from build123d import *

# Parameters (mm, degrees)
F0_W      = 43.450012
F0_H      = 38.1
F0_R      = 1.6
F1_DEPTH  = 8.5
F2_R      = 2.55
F3_DEPTH  = 3.2
F4_R      = 3.75
F5_DEPTH  = 8.5
F6_W      = 8.75
F6_H      = 8.75
F7_DEPTH  = 6.9
F8_W      = 25
F8_H      = 26
F9_DEPTH  = 5
F10_W     = 22
F10_H     = 3
F11_DEPTH = 9.225006


with BuildPart() as f1:
    # F0 (on Top) → F1 (new body)
    with BuildSketch(Plane.XY):
        Rectangle(F0_W, F0_H)
        with Locations((-15.875, -15.875)):
            Circle(F0_R, mode=Mode.SUBTRACT)
        with Locations((15.875, -15.875)):
            Circle(F0_R, mode=Mode.SUBTRACT)
        with Locations((-15.875, 15.875)):
            Circle(F0_R, mode=Mode.SUBTRACT)
        with Locations((15.875, 15.875)):
            Circle(F0_R, mode=Mode.SUBTRACT)
    extrude(amount=F1_DEPTH)

    # F2 (on face) → F3 (cut)
    with BuildSketch(Plane.XY.offset(8.5)):
        with Locations((-15.875, 15.875)):
            Circle(F2_R)
        with Locations((-15.875, -15.875)):
            Circle(F2_R)
        with Locations((15.875, 15.875)):
            Circle(F2_R)
        with Locations((15.875, -15.875)):
            Circle(F2_R)
    extrude(amount=-F3_DEPTH, mode=Mode.SUBTRACT)

    # F4 (on face) → F5 (cut, through all)
    with BuildSketch(Plane.XY.offset(8.5)):
        with Locations((-1.274994, 0)):
            Circle(F4_R)
    extrude(amount=-F5_DEPTH, mode=Mode.SUBTRACT)

    # F6 (on face) → F7 (cut)
    with BuildSketch(Plane(origin=(0, 0, 0), x_dir=(1, 0, 0), z_dir=(0, 0, -1))):
        with Locations((-1.274994, 0)):
            Rectangle(F6_W, F6_H)
    extrude(amount=-F7_DEPTH, mode=Mode.SUBTRACT)

    # F8 (on face) → F9 (cut)
    with BuildSketch(Plane(origin=(0, 0, 0), x_dir=(1, 0, 0), z_dir=(0, 0, -1))):
        Rectangle(F8_W, F8_H)
    extrude(amount=-F9_DEPTH, mode=Mode.SUBTRACT)

    # F10 (on face) → F11 (cut, through all)
    with BuildSketch(Plane(origin=(-21.725006, 0, 0), x_dir=(0, -1, 0), z_dir=(-1, 0, 0))):
        with Locations((0, 1.5)):
            Rectangle(F10_W, F10_H)
    extrude(amount=-F11_DEPTH, mode=Mode.SUBTRACT)


solid = f1.part
The model under review builds one solid part; all positions refer to its coordinate system, in mm. A direction names the side the tool comes from. Coordinates: 2 decimals unless noted, no trailing zeros. Write each loop counter-clockwise with the first axis right and the second up, starting at its lowest first coordinate (ties: lowest second). Pieces come first, ordered by that corner, then holes. Notation, with made-up numbers: (88.5, 69) - (125.5, 69) arc R22 ccw to (125.5, 88) - close; hole circle Ø9 at (50.5, 58.25). An arc over 180 degrees is marked (long way). Answer as a JSON object with one key per item and string values. Group by question number.
1. Add section A-A (y = 0). Give the boundary of the cut face in (x, z) (3 decimals).
2. Add section C-C (y = -15). Give the boundary of the cut face in (x, z) (3 decimals).
3. Mouldability with a two-part tool opening along Y and no side actions: class faces 1 (the face through (14, 0, 0)), 2 (the face through (14.277, -15.805, 2.613)), 3 (the face through (-6, 0, 5)), 4 (the face through (0, -19.05, 4)) as pulls with the +Y half, pulls with the -Y half, needs draft (parallel to the pull), parting line crosses it, or undercut.
4. Clearance check with flat-ended pins moving along their axes: pin 1 Ø5.5 at (x, y) = (16, -16) entering from +Z; pin 2 Ø10 at (x, y) = (-10.5, -3) entering from -Z; pin 3 Ø4 at (x, y) = (-15.875, 15.875) entering from +Z; pin 4 Ø2 at (x, y) = (-8.5, -9) entering from -Z. State where each tip first meets the part, or that it passes through.
5. Add section D-D (z = 7.75). Give the boundary of the cut face in (x, y) (3 decimals), plus the area to 3 significant figures.
6. To check wall thickness, follow probe 1 along X at (y, z) = (-7, 4.5) (3 decimals); probe 2 along Y at (x, z) = (-18, 7.25); probe 3 along Y at (x, z) = (14.5, 3.25). State the ranges of each line that lie inside material, in increasing order.
7. Add section B-B (x = -10). Give the boundary of the cut face in (y, z), plus the area to 3 significant figures.
8. Machinability: for faces 5 (the face through (-1, -4.375, 6)), 6 (the face through (-21.725, 0, 5)), 7 (the face through (-17, 11, 1)), 8 (the face through (-17.05, 16.96, 2.61)), 9 (the face through (16, 14, 5.3)), which of the approach directions +Z, -Z, +X, -X, +Y, -Y give a long, thin tool a straight path to every point of the face, cutting with its end or side? Answer none if there is none.
Findings:
{
 "1": {"outline": "(-21.725, 3) - (-12.5, 3) - (-12.5, 5) - (-5.65, 5) - (-5.65, 6.9) - (-5.025, 6.9) - (-5.025, 8.5) - (-21.725, 8.5) - close; (2.475, 6.9) - (3.1, 6.9) - (3.1, 5) - (12.5, 5) - (12.5, 0) - (21.725, 0) - (21.725, 8.5) - (2.475, 8.5) - close"},
 "2": {"outline": "(-21.725, 0) - (-17.215, 0) - (-17.215, 5.3) - (-18.27, 5.3) - (-18.27, 8.5) - (-21.725, 8.5) - close; (-14.535, 0) - (14.535, 0) - (14.535, 5.3) - (13.48, 5.3) - (13.48, 8.5) - (-13.48, 8.5) - (-13.48, 5.3) - (-14.535, 5.3) - close; (17.215, 0) - (21.725, 0) - (21.725, 8.5) - (18.27, 8.5) - (18.27, 5.3) - (17.215, 5.3) - close"},
 "3": {"face 1": "needs draft", "face 2": "undercut", "face 3": "undercut", "face 4": "pulls with the -Y half"},
 "4": {"pin 1": "z = 8.5", "pin 2": "z = 3", "pin 3": "z = 5.3", "pin 4": "z = 5"},
 "5": {"outline": "(-21.725, -19.05) - (21.725, -19.05) - (21.725, 19.05) - (-21.725, 19.05) - close; hole circle Ø5.1 at (-15.875, -15.875); hole circle Ø5.1 at (-15.875, 15.875); hole circle Ø7.5 at (-1.275, 0); hole circle Ø5.1 at (15.875, -15.875); hole circle Ø5.1 at (15.875, 15.875)", "area": "1,530 mm²"},
 "6": {"probe 1": "-21.725 to -12.5, 12.5 to 21.725", "probe 2": "-19.05 to -17.28, -14.47 to 14.47, 17.28 to 19.05", "probe 3": "-19.05 to -16.69, -15.06 to 15.06, 16.69 to 19.05"},
 "7": {"outline": "(-19.05, 0) - (-13, 0) - (-13, 5) - (13, 5) - (13, 0) - (19.05, 0) - (19.05, 8.5) - (-19.05, 8.5) - close", "area": "194 mm²"},
 "8": {"face 5": "-Z", "face 6": "+Z, -Z, -X, +Y, -Y", "face 7": "-Z, -X", "face 8": "+Z, -Z", "face 9": "+Z"}
}
